For this review, take the finished solid that the model builds, in its own axes (mm). A direction names the side the tool comes from. Coordinates: 2 decimals unless noted, no trailing zeros. Write each loop counter-clockwise with the first axis right and the second up, starting at its lowest first coordinate (ties: lowest second). Pieces come first, ordered by that corner, then holes. Notation, with made-up numbers: (80, -9.5) - (91, -9.5) arc R35 ccw to (91, 25.5) - close; hole circle Ø5 at (-12.75, -29.5). An arc over 180 degrees is marked (long way). Write each question's results on one line, items separated by ' | '.
from build123d import *

# Parameters (mm, degrees)
PAD001_DEPTH    = 5.08
PAD_DEPTH       = 0.2625
SKETCH004_W     = 10.16
SKETCH004_H     = 2.54
PAD002_DEPTH    = 14.1
SKETCH005_R     = 1.59
POCKET_DEPTH    = 2.541
POCKET001_DEPTH = 10.161


with BuildPart() as pad001:
    # Sketch001 → Pad001 (new body, symmetric)
    with BuildSketch(Plane.YZ.offset(2.54)):
        Polygon((0, 3.23), (-1.415, 3.73), (-1.415, 11.42), (-0.415, 12.42), (3.285, 12.42), (3.285, 3.73), align=None)
    extrude(amount=PAD001_DEPTH, both=True)


with BuildPart() as pad:
    # Sketch → Pad (new body, symmetric)
    with BuildSketch(Plane.XZ):
        Polygon((-0.6775, 0.2775), (-0.4, 0), (-0.4, -9.05718), (0, -9.75), (0.4, -9.05718), (0.4, 0), (0.6775, 0.2775), (0.6775, 3.73), (-0.6775, 3.73), align=None)
        Polygon((4.4025, 0.2775), (4.68, 0), (4.68, -9.05718), (5.08, -9.75), (5.48, -9.05718), (5.48, 0), (5.7575, 0.2775), (5.7575, 3.73), (4.4025, 3.73), align=None)
    extrude(amount=PAD_DEPTH, both=True)


with BuildPart() as to_220f_2_vertical:
    # Sketch004 → Pad002 (new body)
    with BuildSketch(Plane.XY.offset(5)):
        with Locations((2.54, 2.015)):
            Rectangle(SKETCH004_W, SKETCH004_H)
    extrude(amount=PAD002_DEPTH)

    # Sketch005 → Pocket (cut, through all)
    with BuildSketch(Plane(origin=(0, 0.745, 5), x_dir=(1, 0, 0), z_dir=(0, -1, 0))):
        with Locations((2.54, 10.8)):
            Circle(SKETCH005_R)
    extrude(amount=-POCKET_DEPTH, mode=Mode.SUBTRACT)

    # Sketch006 → Pocket001 (cut, through all)
    with BuildSketch(Plane(origin=(7.62, 0, 5), x_dir=(0, 1, 0), z_dir=(1, 0, 0))):
        Polygon((2.585, 14.1), (0.745, 13.939021), (0.745, 14.939021), (3.285, 14.939021), (3.285, 14.038758), align=None)
    extrude(amount=-POCKET001_DEPTH, mode=Mode.SUBTRACT)

    add(pad001.part)
    add(pad.part)


solid = to_220f_2_vertical.part
Q1. Mouldability with a two-part tool opening along X and no side actions: class faces 5 (the face through (7.62, 1, 10)), 6 (the face through (2.195, 1.997, 14.248)), 7 (the face through (3, 3.285, 11)), 8 (the face through (-2.54, 1, 10)) as pulls with the +X half, pulls with the -X half, needs draft (parallel to the pull), parting line crosses it, or undercut.
Results found:
face 5: pulls with the +X half | face 6: undercut | face 7: needs draft | face 8: pulls with the -X half
Q2. Take a section at C-C on y = 2.9. State the section outline as (x, z) points.
Results found:
outline: (-2.54, 3.67) - (7.62, 3.67) - (7.62, 19.07) - (-2.54, 19.07) - close; hole circle Ø3.18 at (2.54, 15.8)
Q3. Take a section at D-D on x = 1.25. State the section outline as (y, z) points (3 decimals), plus the area to 3 significant figures.
Results found:
outline: (-1.415, 3.73) - (0, 3.23) - (3.285, 3.73) - (3.285, 14.87) - (0.745, 14.87) - (0.745, 12.42) - (-0.415, 12.42) - (-1.415, 11.42) - close; (0.745, 16.73) - (3.285, 16.73) - (3.285, 19.039) - (2.585, 19.1) - (0.745, 18.939) - close | area: 53.6 mm2
Q4. For pin 1 (4 mm diameter, centred on x = 2.54, z = 15.8, fed in from +Y) (3 decimals); pin 2 (0.7 mm diameter, centred on x = 0, z = -3, fed in from -Y); pin 3 (2 mm diameter, centred on x = 3.5, z = 16, fed in from -Y) (3 decimals); pin 4 (1.3 mm diameter, centred on x = 2.5, y = 0.5, fed in from +Z), all flat-tipped, find the tip position at first contact; note any pin that passes through.
Results found:
pin 1: y = 3.285 | pin 2: y = -0.26 | pin 3: y = 0.745 | pin 4: z = 18.97
Q5. Take a section at B-B on x = 2.54. State the section outline as (y, z) points (3 decimals).
Results found:
outline: (-1.415, 3.73) - (0, 3.23) - (3.285, 3.73) - (3.285, 14.21) - (0.745, 14.21) - (0.745, 12.42) - (-0.415, 12.42) - (-1.415, 11.42) - close; (0.745, 17.39) - (3.285, 17.39) - (3.285, 19.039) - (2.585, 19.1) - (0.745, 18.939) - close
Q6. Take a section at A-A on z = 15.8. State the section outline as (x, y) points (3 decimals).
Results found:
outline: (-2.54, 0.745) - (0.95, 0.745) - (0.95, 3.285) - (-2.54, 3.285) - close; (4.13, 0.745) - (7.62, 0.745) - (7.62, 3.285) - (4.13, 3.285) - close
Q7. Wall thickness on line 1 along Y through (x, z) = (0.25, -4.5); line 2 along Y through (x, z) = (-0.75, 17.25) (3 decimals); line 3 along Z through (x, y) = (2.54, 2.6): over which ranges is each line inside the solid? List them lowest first. Write a range as from..to.
Results found:
line 1: -0.26..0.26 | line 2: 0.745..3.285 | line 3: 3.63..14.21, 17.39..19.1
Q8. For faces 1 (the face through (3, 0, 12.42)), 2 (the face through (3, -1.415, 8)), 3 (the face through (5, -0.262, -2)), 4 (the face through (0, 0.262, -2)), list the 3-axis set-ups (+Z, -Z, +X, -X, +Y, -Y) from which the entire face can be reached by the end or side of a thin tool; tool diameter is ignored.
Results found:
face 1: +Z, +X, -X, -Y | face 2: +Z, -Z, +X, -X, -Y | face 3: -Z, +X, -X, -Y | face 4: -Z, +X, -X, +Y
